```python
from build123d import *

# Parameters (mm, degrees)
BOSS_EXTRUDE1_DEPTH = 25
CUT_EXTRUDE3_START  = -25
SKETCH5_R           = 4.4
CUT_EXTRUDE3_DEPTH  = 4.5
SKETCH6_OUTSIDE_W   = 108.03
SKETCH6_OUTSIDE_H   = 47.53
CUT_EXTRUDE4_DEPTH  = 25
SKETCH8_W           = 50.5
SKETCH8_H           = 25.070079704
CUT_EXTRUDE5_DEPTH  = 3.5


with BuildPart() as part:
    # Sketch2 → Boss-Extrude1 (new body)
    with BuildSketch(Plane.XY):
        with BuildLine():
            Line((53.900497512, 28.014925373), (27.014667046, 28.014925373))
            ThreePointArc((27.014667046, 28.014925373), (25.389308303, 27.180347595), (25.120437848, 25.373134328))
            ThreePointArc((25.120437848, 25.373134328), (11.150497512, 5.889925373), (-2.819442823, 25.373134328))
            ThreePointArc((-2.819442823, 25.373134328), (-3.088313278, 27.180347595), (-4.713672021, 28.014925373))
            Line((-4.713672021, 28.014925373), (-31.599502488, 28.014925373))
            Line((-31.599502488, 28.014925373), (-31.599502488, -22.985074627))
            Line((-31.599502488, -22.985074627), (53.900497512, -22.985074627))
            Line((53.900497512, -22.985074627), (53.900497512, 28.014925373))
        make_face()
    extrude(amount=BOSS_EXTRUDE1_DEPTH)

    # Sketch5 → Cut-Extrude3 (cut)
    with BuildSketch(Plane.XY.offset(25).offset(CUT_EXTRUDE3_START)):
        with Locations((11.150497512, -2.910074627)):
            Circle(SKETCH5_R)
    extrude(amount=CUT_EXTRUDE3_DEPTH, mode=Mode.SUBTRACT)

    # Sketch6 outside → Cut-Extrude4 (cut)
    with BuildSketch(Plane(origin=(0, 28.014925373, 0), x_dir=(1, 0, 0), z_dir=(0, 1, 0))):
        with Locations((11.15, -12.5)):
            Rectangle(SKETCH6_OUTSIDE_W, SKETCH6_OUTSIDE_H)
        Polygon((-24.599502488, 0), (-26.73851519, -7.13632431), (-14.574659319, -7.13632431), (-16.713672021, 0), (-4.713672021, 0), (27.014667046, 0), (39.014667046, 0), (36.875076634, -7.136151124), (49.040087925, -7.136151124), (46.900497512, 0), (53.900497512, 0), (53.900497512, -25), (46.900497512, -25), (49.040087925, -17.863848876), (36.875076634, -17.863848876), (39.014667046, -25), (27.014667046, -25), (-4.713672021, -25), (-16.713672021, -25), (-14.574081609, -17.863848876), (-26.7390929, -17.863848876), (-24.599502488, -25), (-31.599502488, -25), (-31.599502488, 0), align=None, mode=Mode.SUBTRACT)
    extrude(amount=-CUT_EXTRUDE4_DEPTH, mode=Mode.SUBTRACT)

    # Sketch8 → Cut-Extrude5 (cut)
    with BuildSketch(Plane(origin=(0, 0, 2.5), x_dir=(-1, 0, 0), z_dir=(0, 0, -1))):
        with Locations((-11.150497512, 15.479885521)):
            Rectangle(SKETCH8_W, SKETCH8_H)
    extrude(amount=-CUT_EXTRUDE5_DEPTH, mode=Mode.SUBTRACT)


solid = part.part
```
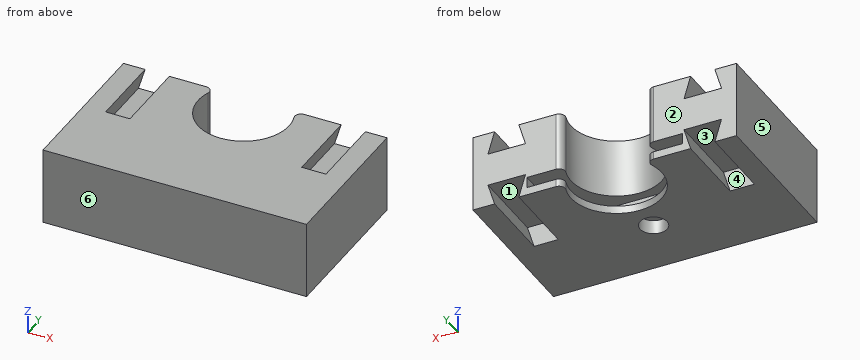
The listing builds one solid part. Answer for the finished solid, in the listing's coordinates (mm). Face numbers are marked on the shaded views. A direction names the side the tool comes from. Coordinates: 2 decimals unless noted, no trailing zeros. Loops run counter-clockwise (first coordinate to the right, second up) from the corner with the lowest first, then second, coordinate; pieces in that order, holes last. Notation, with made-up numbers: (68, -35.5) -> (116, -35.5) arc R18 cw to (116, -8.5) -> close; hole circle Ø10 at (42, -3). An arc over 180 degrees is marked (long way). Return JSON: item names as keys, results as strings. Group by question number.
(1) Given pin 1 Ø7 at (x, y) = (11.15, -2.91) entering from -Z; pin 2 Ø20 at (x, y) = (13, 21.5) entering from -Z; pin 3 Ø3.5 at (x, z) = (42, 21) entering from +Y; pin 4 Ø1 at (x, z) = (20, 4.5) entering from +Y, each flat-ended and moving along its own axis, determine where each tip first touches the part or whether it passes through.
(2) Determine the mould class of the marked faces 3, 4, 5 and 6 for opening direction X: released by +X, released by -X, zero draft, split by the parting line, or undercut.
(3) A cutting plane is placed at A-A on x = 35. Write down the section's boundary in (y, z).
(4) A cutting plane is placed at C-C on z = 20. Write down the section's boundary in (x, y).
(5) Which of the six approach directions +Z, -Z, +X, -X, +Y, -Y give full straight-line access (tool end or side, diameter ignored) to the marked faces 1 and 2?
(6) Find the intervals of material crossed by probe 1 along Z at (x, y) = (-8, 15.5); probe 2 along X at (y, z) = (10, 5.5); probe 3 along X at (y, z) = (15, 7), in increasing order. Write a range as from..to.
The answers:
{
 "1": {"pin 1": "stops at z = 4.5", "pin 2": "passes through", "pin 3": "stops at y = 3.01", "pin 4": "stops at y = 2.94"},
 "2": {"face 3": "undercut", "face 4": "undercut", "face 5": "released by -X", "face 6": "zero draft"},
 "3": {"outline": "(-22.99, 0) -> (28.01, 0) -> (28.01, 2.5) -> (2.94, 2.5) -> (2.94, 6) -> (28.01, 6) -> (28.01, 25) -> (-22.99, 25) -> close"},
 "4": {"outline": "(-31.6, -22.99) -> (53.9, -22.99) -> (53.9, 28.01) -> (48.4, 28.01) -> (48.4, 3.01) -> (37.52, 3.01) -> (37.52, 28.01) -> (27.01, 28.01) arc R2 ccw to (25.12, 25.37) arc R14.75 cw (long way) to (-2.82, 25.37) arc R2 ccw to (-4.71, 28.01) -> (-15.21, 28.01) -> (-15.21, 3.01) -> (-26.1, 3.01) -> (-26.1, 28.01) -> (-31.6, 28.01) -> close"},
 "5": {"face 1": "+Y", "face 2": "+Z, -Z, +X, -X, +Y"},
 "6": {"probe 1": "z = 0..2.5, 6..25", "probe 2": "x = -31.6..-26.25, -15.07..-14.1, 36.4..37.37, 48.55..53.9", "probe 3": "x = -31.6..-26.7, -14.62..-2.48, 24.78..36.92, 49..53.9"}
}
